Input: part model. Units: mm. Frame: model coordinates. A direction names the side the tool comes from. Give positions to 0.01 mm unless a question says otherwise; leave off trailing zeros. Loops run counter-clockwise (first coordinate to the right, second up) from the corner with the lowest first, then second, coordinate; pieces in that order, holes last. Notation, with made-up numbers: (-21.5, -38) -> (-7.5, -38) arc R26 cw to (-7.5, -2) -> close; hole circle Ø7 at (-11.75, -15). An arc over 180 degrees is marked (long way). Answer as a JSON object with one key per item and string values.
```python
from build123d import *

# Parameters (mm, degrees)
BOSS_EXTRUDE1_DEPTH = 19.05
FILLET1_R           = 6.35
CUT_EXTRUDE1_DEPTH  = 7.5


with BuildPart() as part:
    # Sketch1 → Boss-Extrude1 (new body)
    with BuildSketch(Plane(origin=(0, 0, 0), x_dir=(1, 0, 0), z_dir=(0, 1, 0))):
        Polygon((0, 38.1), (-6.35, 0), (-6.35, -19.685), (6.35, -19.685), (6.35, 0), align=None)
    extrude(amount=BOSS_EXTRUDE1_DEPTH)

    # Fillet1
    fillet1_edges = [part.edges().sort_by_distance(p)[0] for p in [
        (-6.35, 9.525, 19.685),
        (6.35, 9.525, 19.685),
    ]]
    fillet(fillet1_edges, radius=FILLET1_R - 0.0001)  # a hair under: the kernel refuses the full size

    # Sketch4 → Cut-Extrude1 (cut)
    with BuildSketch(Plane(origin=(0, 19.05, 0), x_dir=(1, 0, 0), z_dir=(0, 1, 0))):
        with BuildLine():
            Line((-4.831855252, -13.202514523), (-3.088402326, 6.896250909))
            ThreePointArc((-3.088402326, 6.896250909), (0, 9.728349675), (3.088402326, 6.896250909))
            Line((3.088402326, 6.896250909), (4.831855252, -13.202514523))
            ThreePointArc((4.831855252, -13.202514523), (0, -18.471650325), (-4.831855252, -13.202514523))
        make_face()
    extrude(amount=-CUT_EXTRUDE1_DEPTH, mode=Mode.SUBTRACT)


solid = part.part
```
Q1. Ray query, line 1 along Y through (x, z) = (-3.5, 7); line 2 along X through (y, z) = (15.75, 6); line 3 along X through (y, z) = (15.25, 17). Return the intervals inside material, ascending.
Evaluation:
{"line 1": "y = 0 to 11.55", "line 2": "x = -6.35 to -4.21, 4.21 to 6.35", "line 3": "x = -5.19 to -3.48, 3.48 to 5.19"}
Q2. Section D-D, the plane x = -2. Return the cut outline in (y, z), then the cut area to 3 significant figures.
Evaluation:
{"outline": "(0, -26.1) -> (19.05, -26.1) -> (19.05, -9) -> (11.55, -9) -> (11.55, 18.04) -> (19.05, 18.04) -> (19.05, 19.36) -> (0, 19.36) -> close", "area": "663 mm2"}
Q3. Draft query along X for faces 3 (the flat face through (-3.97, 15.35, 3.29)), 4 (the flat face through (0, 0, -3)), 5 (the cylindrical face through (-4.539, 9.658, 17.776)). Return one class per face: +X half, -X half, draft (parallel to the pull), parting line (faces both ways), or undercut.
Evaluation:
{"face 3": "undercut", "face 4": "draft", "face 5": "-X half"}
Q4. Section C-C, the plane z = 12.5. Return the cut outline in (x, y), then the cut area to 3 significant figures.
Evaluation:
{"outline": "(-6.35, 0) -> (6.35, 0) -> (6.35, 19.05) -> (4.77, 19.05) -> (4.77, 11.55) -> (-4.77, 11.55) -> (-4.77, 19.05) -> (-6.35, 19.05) -> close", "area": "170 mm2"}
Q5. Access query for faces 1 (the cylindrical face through (4.441, 9.658, 17.874)), 2 (the flat face through (0, 11.55, 4)). Directions: +Z, -Z, +X, -X, +Y, -Y. A direction counts if a zero-diameter tool reaches every point of the face in a straight line with its end or side. Return the directions, or none.
Evaluation:
{"face 1": "+Z, +X, +Y, -Y", "face 2": "+Y"}
Q6. Pin query (flat end, axial travel): pin 1 (3 mm diameter, centred on y = 12.5, z = -7.5, fed in from +X); pin 2 (4 mm diameter, centred on y = 7, z = -4, fed in from -X); pin 3 (10 mm diameter, centred on y = 15.5, z = -19.5, fed in from +X). Return the tip coordinate at first contact, or that it passes through.
Evaluation:
{"pin 1": "stops at x = 5.35", "pin 2": "stops at x = -6.02", "pin 3": "stops at x = 3.93"}
